```python
from build123d import *

# Parameters (mm, degrees)
SKETCH1_R           = 9.525
SKETCH1_R_2         = 4.7625
BOSS_EXTRUDE1_DEPTH = 15.875
BOSS_EXTRUDE2_START = 15.875
SKETCH1_3_R         = 15.875
SKETCH1_3_R_2       = 4.7625
BOSS_EXTRUDE2_DEPTH = 3.175


with BuildPart() as part:
    # Sketch1 → Boss-Extrude1 (new body)
    with BuildSketch(Plane.XY):
        Circle(SKETCH1_R)
        Circle(SKETCH1_R_2, mode=Mode.SUBTRACT)
    extrude(amount=BOSS_EXTRUDE1_DEPTH)

    # Sketch1<3> → Boss-Extrude2 (add)
    with BuildSketch(Plane.XY.offset(BOSS_EXTRUDE2_START)):
        Circle(SKETCH1_3_R)
        Circle(SKETCH1_3_R_2, mode=Mode.SUBTRACT)
    extrude(amount=BOSS_EXTRUDE2_DEPTH)

    # Mirror1: part across plane


with BuildPart() as part_1:
    add(part.part)
    add(part.part.mirror(Plane.XY))


solid = part_1.part
```
Work out the finished part from the listing and answer in its coordinate system (mm). A direction names the side the tool comes from. Give positions to 0.01 mm unless a question says otherwise; leave off trailing zeros. Order: outer loops, then holes, each group sorted by start corner. A loop starts at its lowest first (then second) coordinate and runs counter-clockwise, first axis right, second up. Notation, with made-up numbers: (-14.75, 15) -> (16.25, 15) arc R20 ccw to (16.25, 49) -> close; hole circle Ø10 at (2, 29). An arc over 180 degrees is marked (long way). Answer as CSV lines item,"result". Start each with the question number.
(1) Each of these flat-tipped pins is pushed along its axis until it touches: pin 1 Ø15 at (x, y) = (0, 0) entering from +Z; pin 2 Ø5 at (x, z) = (-8, 9) entering from +Y; pin 3 Ø3 at (x, z) = (6.5, -6) entering from +Y; pin 4 Ø2 at (y, z) = (-8, 3) entering from +X. Where does it stop, or does it pass through?
(2) Consider line 1 along Y through (x, z) = (0, 8.5) (1 decimal); line 2 along Z through (x, y) = (7, 7) (3 decimals); line 3 along Y through (x, z) = (3, 0). Determine where each line is inside the solid, lowest interval first.
(3) Section D-D, the plane y = 9 is taken. Write down the section's boundary in (x, z) (3 decimals), plus the area to 3 significant figures.
(4) Which of the six approach directions +Z, -Z, +X, -X, +Y, -Y give full straight-line access (tool end or side, diameter ignored) to faces 1 (the flat face through (3, 4, -19.05)), 2 (the cylindrical face through (-7.559, -5.796, 0.222))?
(5) For a pull along X with two mould halves and no side action, classify faces 3 (the cylindrical face through (-3.78, -2.9, 0.27)), 4 (the flat face through (7, -7, -15.875)), 5 (the cylindrical face through (-3.441, -15.497, 17.44)) as released by +X, released by -X, zero draft, split by the parting line, or undercut.
Entries:
1,pin 1,"z = 19.05"
1,pin 2,"y = 7.78"
1,pin 3,"y = 8.11"
1,pin 4,"x = 6.46"
2,line 1,"-9.5 to -4.8, 4.8 to 9.5"
2,line 2,"-19.05 to -15.875, 15.875 to 19.05"
2,line 3,"-9.04 to -3.7, 3.7 to 9.04"
3,outline,"(-13.077, -19.05) -> (13.077, -19.05) -> (13.077, -15.875) -> (3.119, -15.875) -> (3.119, 15.875) -> (13.077, 15.875) -> (13.077, 19.05) -> (-13.077, 19.05) -> (-13.077, 15.875) -> (-3.119, 15.875) -> (-3.119, -15.875) -> (-13.077, -15.875) -> close"
3,area,"364 mm²"
4,face 1,"-Z, +X, -X, +Y, -Y"
4,face 2,"none"
5,face 3,"undercut"
5,face 4,"zero draft"
5,face 5,"split by the parting line"
